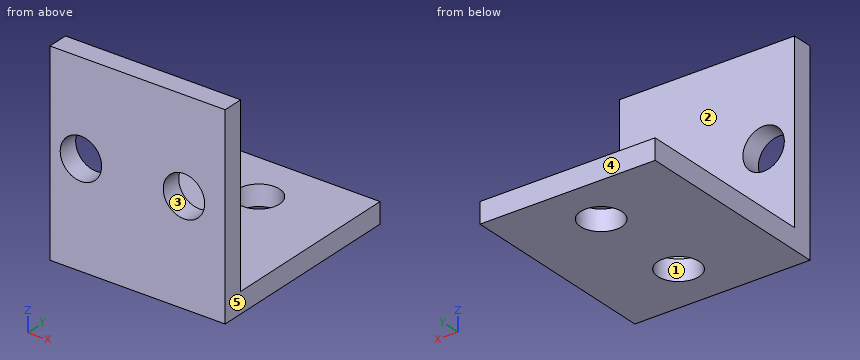
from build123d import *

# Parameters (mm, degrees)
SKETCH1_W           = 21.59
SKETCH1_H           = 25.4
BOSS_EXTRUDE1_DEPTH = 24.13
SKETCH2_W           = 21.59
SKETCH2_H           = 22.86
CUT_EXTRUDE1_DEPTH  = 42.152703435
SKETCH3_R           = 2.5527
CUT_EXTRUDE2_DEPTH  = 40.716699259
SKETCH4_R           = 2.5527
CUT_EXTRUDE3_DEPTH  = 40.635395797


with BuildPart() as part:
    # Sketch1 → Boss-Extrude1 (new body)
    with BuildSketch(Plane.XY):
        with Locations((10.795, 12.7)):
            Rectangle(SKETCH1_W, SKETCH1_H)
    extrude(amount=BOSS_EXTRUDE1_DEPTH)

    # Sketch2 → Cut-Extrude1 (cut, through all)
    with BuildSketch(Plane(origin=(21.59, 0, 0), x_dir=(0, 0, -1), z_dir=(1, 0, 0))):
        with Locations((-13.335, 13.97)):
            Rectangle(SKETCH2_W, SKETCH2_H)
    extrude(amount=-CUT_EXTRUDE1_DEPTH, mode=Mode.SUBTRACT)

    # Sketch3 → Cut-Extrude2 (cut, through all)
    with BuildSketch(Plane.XY.offset(2.54)):
        with Locations((11.43, 19.05)):
            Circle(SKETCH3_R)
        with Locations((11.43, 6.35)):
            Circle(SKETCH3_R)
    extrude(amount=-CUT_EXTRUDE2_DEPTH, mode=Mode.SUBTRACT)

    # Sketch4 → Cut-Extrude3 (cut, through all)
    with BuildSketch(Plane(origin=(0, 2.54, 0), x_dir=(1, 0, 0), z_dir=(0, 1, 0))):
        with Locations(Location((16.51, -12.7, 0), (0, 0, 270))):
            Circle(SKETCH4_R)
        with Locations(Location((3.81, -12.7, 0), (0, 0, 270))):
            Circle(SKETCH4_R)
    extrude(amount=-CUT_EXTRUDE3_DEPTH, mode=Mode.SUBTRACT)


solid = part.part
Can you work these out from the model? Positions are in its coordinate system, mm. Face numbers are marked on the shaded views. A direction names the side the tool comes from. Give positions to 0.01 mm unless a question says otherwise; leave off trailing zeros. Loops run counter-clockwise (first coordinate to the right, second up) from the corner with the lowest first, then second, coordinate; pieces in that order, holes last. Notation, with made-up numbers: (52.25, -33) - (78.25, -33) arc R6 ccw to (78.25, -29) - close; hole circle Ø1 at (-8.75, -4.5). An arc over 180 degrees is marked (long way). Answer as a JSON object with one key per item and string values.
Q1. Imagine slicing it at D-D on x = 11.43. Write out the boundary of the cut face in (y, z), plus the area to 3 significant figures.
Geometry says:
{"outline": "(0, 0) - (3.8, 0) - (3.8, 2.54) - (2.54, 2.54) - (2.54, 24.13) - (0, 24.13) - close; (8.9, 0) - (16.5, 0) - (16.5, 2.54) - (8.9, 2.54) - close; (21.6, 0) - (25.4, 0) - (25.4, 2.54) - (21.6, 2.54) - close", "area": "93.4 mm²"}
Q2. Imagine slicing it at C-C on z = 12.7. Write out the boundary of the cut face in (x, y), plus the area to 3 significant figures.
Geometry says:
{"outline": "(0, 0) - (1.26, 0) - (1.26, 2.54) - (0, 2.54) - close; (6.36, 0) - (13.96, 0) - (13.96, 2.54) - (6.36, 2.54) - close; (19.06, 0) - (21.59, 0) - (21.59, 2.54) - (19.06, 2.54) - close", "area": "28.9 mm²"}
Q3. Imagine slicing it at B-B on x = 3.81. Write out the boundary of the cut face in (y, z).
Geometry says:
{"outline": "(0, 0) - (25.4, 0) - (25.4, 2.54) - (2.54, 2.54) - (2.54, 10.15) - (0, 10.15) - close; (0, 15.25) - (2.54, 15.25) - (2.54, 24.13) - (0, 24.13) - close"}
Q4. Imagine slicing it at A-A on y = 19.05. Write out the boundary of the cut face in (x, z).
Geometry says:
{"outline": "(0, 0) - (8.88, 0) - (8.88, 2.54) - (0, 2.54) - close; (13.98, 0) - (21.59, 0) - (21.59, 2.54) - (13.98, 2.54) - close"}
Q5. If we mould it in two halves opening along X, with no side actions, what happens to the marked faces 3, 4 and 5? For each: pulls with the +X half, pulls with the -X half, needs draft (parallel to the pull), parting line crosses it, or undercut.
Geometry says:
{"face 3": "undercut", "face 4": "needs draft", "face 5": "pulls with the +X half"}
Q6. Will these pins go through, and if not, where does the flat tip stop? P1, Ø8, axis at y = 19.5, z = 8, coming from the +X side; P2, Ø6.5, axis at x = 16.51, z = 12.7, coming from the +Y side; P3, Ø8, axis at x = 5.5, y = 7, coming from the +Z side.
Geometry says:
{"P1": "through", "P2": "y = 2.54", "P3": "z = 2.54"}
Q7. If I drill on L1, parallel to X at y = 0.55, z = 12.7; L2, parallel to Y at x = 11.43, z = 1; L3, parallel to Y at x = 2.75, z = 18.5, over which ranges is the centre line in solid material (lowest first)?
Geometry says:
{"L1": "0 to 1.26, 6.36 to 13.96, 19.06 to 21.59", "L2": "0 to 3.8, 8.9 to 16.5, 21.6 to 25.4", "L3": "0 to 2.54"}
Q8. Which directions (+Z, -Z, +X, -X, +Y, -Y) give clear straight access to the entire face, cutting with the end or side of a thin tool? Please do the marked faces 1 and 2.
Geometry says:
{"face 1": "+Z, -Z", "face 2": "+Z, +X, -X, +Y"}
